Verification items for this drawing (mm, ordinates from the low corner). A direction names the side the tool comes from. Round coordinates to 2 decimals unless told otherwise and drop trailing zeros. Loops run counter-clockwise (first coordinate to the right, second up) from the corner with the lowest first, then second, coordinate; pieces in that order, holes last. Notation, with made-up numbers: (-13, -2.5) - (18, -2.5) arc R18 cw to (18, 22.5) - close; hole circle Ø9 at (-16, 81.25). An arc over 180 degrees is marked (long way). Answer in a Markdown table with one row per item. Add a question column.
(1) Cross-section at A-A on x = 5.25. Enter the section's corners in (y, z) (1 decimal), then the cut area to 3 significant figures.
(2) Gauge pin test, flat ends, axial feed: pin 1 (3 mm diameter, centred on x = 6.5, y = 133, fed in from -Z); pin 2 (2 mm diameter, centred on y = 141.5, z = 2, fed in from +X); pin 3 (1.5 mm diameter, centred on y = 37.5, z = 5.5, fed in from -X). Record the tip position at first contact, or that the pin passes through.
(3) Access from +Z, -Z, +X, -X, +Y, -Y to the whole of each face (thin tool, end or side, straight path). Record for the marked faces 1 and 2.
(4) Thickness scan on line 1 along Y through (x, z) = (3, 10) (1 decimal); line 2 along Z through (x, y) = (6.75, 40); line 3 along X through (y, z) = (137, 5.75) (1 decimal). Record the ranges inside material, lowest first.
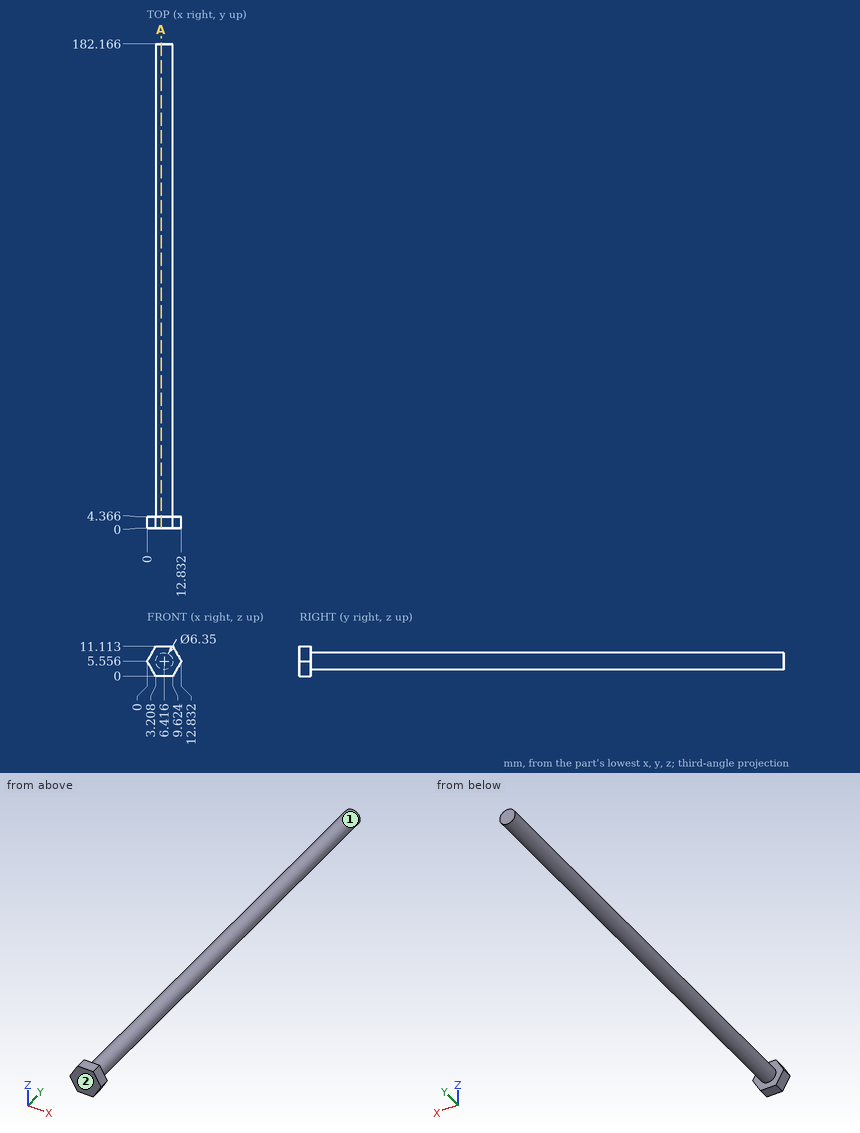
Answers:
| question | item | result |
|---|---|---|
| 1 | outline | (0, 0) - (4.4, 0) - (4.4, 2.6) - (182.2, 2.6) - (182.2, 8.5) - (4.4, 8.5) - (4.4, 11.1) - (0, 11.1) - close |
| 1 | area | 1,100 mm^2 |
| 2 | pin 1 | stops at z = 2.38 |
| 2 | pin 2 | stops at x = 8.3 |
| 2 | pin 3 | stops at x = 3.24 |
| 3 | face 1 | +Y |
| 3 | face 2 | +Z, -Z, +X, -X, -Y |
| 4 | line 1 | y = 0 to 4.4 |
| 4 | line 2 | z = 2.4 to 8.71 |
| 4 | line 3 | x = 3.2 to 9.6 |
